Here's how the part is built. I have some questions about the finished solid (model axes, mm). A direction names the side the tool comes from. Coordinates: 2 decimals unless noted, no trailing zeros. Loops run counter-clockwise (first coordinate to the right, second up) from the corner with the lowest first, then second, coordinate; pieces in that order, holes last. Notation, with made-up numbers: M 63,30.5 L 119,30.5 A34 cw 119,67.5 Z; hole C 34,20.25 d9. An arc over 180 degrees is marked long. Use one line per item in the form item = value. Start each with the question number.
(1) Thinking about a two-plate mould opening in Z: for faces 3 (the flat face through (0, 0, 0)), 4 (the cylindrical face through (-22.63, 0.01, 8.99)), 5 (the flat face through (2, 0, 5)), 6 (the flat face through (-6, -0.75, 3)), which applies, +Z half, -Z half, draft (parallel to the pull), parting line (faces both ways), or undercut?
(2) On a 3-axis mill with a long thin cutter (end or side, diameter ignored), from which of +Z, -Z, +X, -X, +Y, -Y can I reach the whole of each face in a straight line? I mean faces 1 (the flat face through (-20, 0, 6)), 2 (the flat face through (-6, 0.75, 3)). Say none if no direction works.
(3) Imagine slicing it at A-A, the plane y = -0.35. Please give me the cut outline in (x, z), and give its area (3 significant figures).
(4) Imagine slicing it at B-B, the plane x = 15. Please give me the cut outline in (y, z).
(5) Will these pins go through, and if not, where does the flat tip stop? P1, Ø5, axis at x = -5, z = 8, coming from the -Y side; P2, Ø0.8, axis at x = 1.5, y = 0.5, coming from the +Z side.
(6) Please list where these lines run through material, in increasing order: L1, parallel to Z at x = 22.5, y = -0.35; L2, parallel to Z at x = -22.5, y = 0.05; L3, parallel to Z at x = -5, y = -0.4.
```python
from build123d import *

# Parameters (mm, degrees)
F0_R     = 1
F1_DEPTH = 0.75


with BuildPart() as f1:
    # F0 (on Front) → F1 (new body, symmetric)
    with BuildSketch(Plane.XZ):
        with BuildLine():
            Line((-22.5, 0), (0, 0))
            Line((0, 0), (22.5, 0))
            ThreePointArc((22.5, 0), (24.267767, 0.732233), (25, 2.5))
            ThreePointArc((25, 2.5), (24.267767, 4.267767), (22.5, 5))
            Line((22.5, 5), (0, 5))
            Line((0, 5), (-20, 5))
            Line((-20, 5), (-20, 8))
            ThreePointArc((-20, 8), (-20.732233, 9.767767), (-22.5, 10.5))
            ThreePointArc((-22.5, 10.5), (-24.267767, 9.767767), (-25, 8))
            Line((-25, 8), (-25, 2.5))
            ThreePointArc((-25, 2.5), (-24.267767, 0.732233), (-22.5, 0))
        make_face()
        with Locations((22.5, 2.5)):
            Circle(F0_R, mode=Mode.SUBTRACT)
        with Locations((-22.5, 8)):
            Circle(F0_R, mode=Mode.SUBTRACT)
    extrude(amount=F1_DEPTH, both=True)


solid = f1.part
```
Answer:
q1.face_3 = -Z half
q1.face_4 = undercut
q1.face_5 = +Z half
q1.face_6 = draft
q2.face_1 = +Z, +X, +Y, -Y
q2.face_2 = +Z, -Z, +X, -X, +Y
q3.outline = M -25,2.5 A2.5 ccw -22.5,0 L 22.5,0 A2.5 ccw 22.5,5 L -20,5 L -20,8 A2.5 ccw -25,8 Z; hole C -22.5,8 d2; hole C 22.5,2.5 d2
q3.area = 265 mm²
q4.outline = M -0.75,0 L 0.75,0 L 0.75,5 L -0.75,5 Z
q5.P1 = through
q5.P2 = 5
q6.L1 = 0 to 1.5, 3.5 to 5
q6.L2 = 0 to 7, 9 to 10.5
q6.L3 = 0 to 5
